For this review, use the dimensioned drawing (mm, ordinates from the lowest corner) and the shaded views. A direction names the side the tool comes from. Give positions to 0.01 mm unless a question says otherwise; leave off trailing zeros. Loops run counter-clockwise (first coordinate to the right, second up) from the corner with the lowest first, then second, coordinate; pieces in that order, holes last. Notation, with made-up numbers: (22, 8.5) - (52, 8.5) arc R6 cw to (52, 13.5) - close; hole circle Ø7 at (-28, -29). An arc over 180 degrees is marked (long way). Put each result on its own line as item: value.
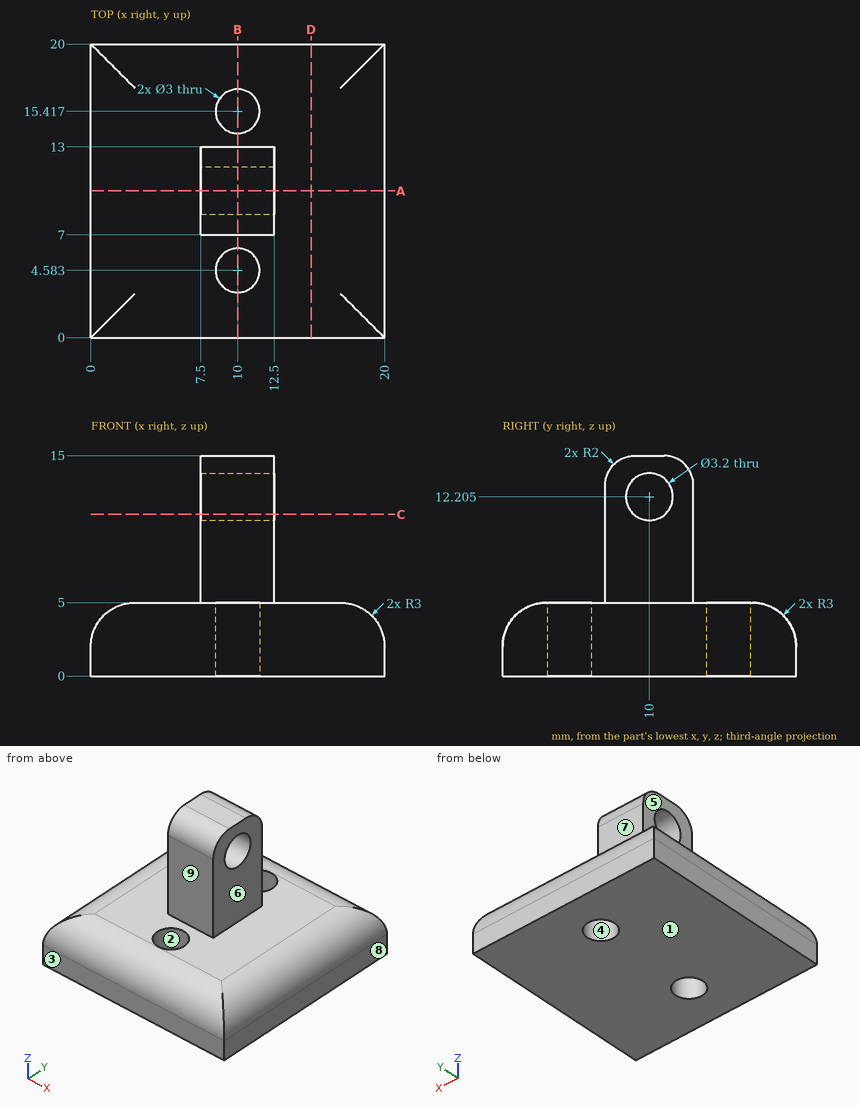
1) Take a section at C-C on z = 11. State the section outline as (x, y) points.
Geometry check:
outline: (7.5, 7) - (12.5, 7) - (12.5, 8.95) - (7.5, 8.95) - close; (7.5, 11.05) - (12.5, 11.05) - (12.5, 13) - (7.5, 13) - close
2) For the marked faces 5, 6, 7, 8 and 9, list the 3-axis set-ups (+Z, -Z, +X, -X, +Y, -Y) from which the entire face can be reached by the end or side of a thin tool; tool diameter is ignored.
Geometry check:
face 5: +Z, -X, +Y, -Y
face 6: +Z, +X, +Y, -Y
face 7: +Z, +X, -X, +Y
face 8: +Z, -Z, +X, +Y, -Y
face 9: +Z, +X, -X, -Y
3) Take a section at A-A on y = 10. State the section outline as (x, z) points (1 decimal), and give its area (3 significant figures).
Geometry check:
outline: (0, 0) - (20, 0) - (20, 2) arc R3 ccw to (17, 5) - (12.5, 5) - (12.5, 10.6) - (7.5, 10.6) - (7.5, 5) - (3, 5) arc R3 ccw to (0, 2) - close; (7.5, 13.8) - (12.5, 13.8) - (12.5, 15) - (7.5, 15) - close
area: 130 mm²
4) Wall thickness on line 1 (Y direction, x = 10, z = 1.55); line 2 (Z direction, x = 8.6, y = 10) (1 decimal); line 3 (Z direction, x = 5.75, y = 14.5): over which ranges is each line inside the solid? List them lowest first.
Geometry check:
line 1: y = 0 to 3.08, 6.08 to 13.92, 16.92 to 20
line 2: z = 0 to 10.6, 13.8 to 15
line 3: z = 0 to 5
5) Take a section at D-D on x = 15. State the section outline as (y, z) points.
Geometry check:
outline: (0, 0) - (20, 0) - (20, 2) arc R3 ccw to (17, 5) - (3, 5) arc R3 ccw to (0, 2) - close
6) Draft analysis for pull direction Y (two halves, no side actions). For the marked faces 1, 2, 3 and 4, state which applies: pulls with the +Y half, pulls with the -Y half, needs draft (parallel to the pull), parting line crosses it, or undercut.
Geometry check:
face 1: needs draft
face 2: undercut
face 3: pulls with the -Y half
face 4: undercut
7) Take a section at B-B on x = 10. State how many separate pieces and enclosed holes the cut face has, and give its area (3 significant figures).
Geometry check:
separate pieces: 3
enclosed holes: 1
area: 116 mm²
8) Insertion check: pin 1 Ø6.5 at (y, z) = (10.5, 12) entering from -X; pin 2 Ø1.5 at (x, z) = (8, 12.5) entering from +Y; pin 3 Ø5 at (x, y) = (7, 6) entering from +Z. Each pin has a flat end and moves straight along its axis. Give the tip position at first contact, or say it passes through.
Geometry check:
pin 1: stops at x = 7.5
pin 2: stops at y = 13
pin 3: stops at z = 14.92
